Read the model definition and answer for the solid it produces. Units are mm, in the model's axes. Round coordinates to 2 decimals unless told otherwise and drop trailing zeros. Order: outer loops, then holes, each group sorted by start corner. A loop starts at its lowest first (then second) coordinate and runs counter-clockwise, first axis right, second up. Notation, with made-up numbers: (49, 68.5) - (103, 68.5) arc R18 cw to (103, 74.5) - close; hole circle Ø11 at (43, 33). An arc over 180 degrees is marked (long way). Answer as a JSON object with one key per item and string values. Group by question number.
Q1. A cutting plane is placed at A-A on y = -17. Determine the outline of the cut face in (x, z).
Q2. A cutting plane is placed at B-B on x = -18. Determine the outline of the cut face in (y, z) (3 decimals).
Q3. A cutting plane is placed at C-C on z = -24. Determine the outline of the cut face in (x, y) (3 decimals), and give its area (3 significant figures).
Q4. Given pin 1 Ø10.5 at (y, z) = (-7.5, 3) entering from +X; pin 2 Ø2.5 at (x, y) = (-34.5, -12) entering from -Z; pin 3 Ø2.5 at (x, y) = (-34, -14.5) entering from +Z, each flat-ended and moving along its own axis, determine where each tip first touches the part or whether it passes through.
Q5. Consider line 1 (Z direction, x = -45.5, y = -2.75); line 2 (Y direction, x = -12, z = 80) (3 decimals); line 3 (X direction, y = -7.5, z = 2). Determine where each line is inside the solid, lowest interval first.
```python
from build123d import *

# Parameters (mm, degrees)
F0_W        = 101.6
F0_H        = 279.4
F1_DEPTH    = 3.175
F2_W        = 3.175
F2_H        = 12.99972
F3_DEPTH    = 16.27124
F2_W_2      = 14.77137
F4_DEPTH    = 25.4
F5_T1_DEPTH = 12.99972
F7_D        = 6.10108


# Not quite as in the source:
# - a fillet or chamfer that OpenCascade refuses, or shapes differently, is made with other operations: its cross-section is extruded or revolved along the edge and cut away or added


with BuildPart() as f1:
    # F0 (on Front) → F1 (new body)
    with BuildSketch(Plane.XZ):
        Rectangle(F0_W, F0_H)
    extrude(amount=F1_DEPTH)

    # F2 (on face) → F3 (join)
    with BuildSketch(Plane.XZ.offset(3.175)):
        with Locations((34.44113, 0)):
            Rectangle(F2_W, F2_H)
        with Locations((-34.44113, 0)):
            Rectangle(F2_W, F2_H)
    extrude(amount=F3_DEPTH)

    # F2 (on face) → F4 (cut)
    with BuildSketch(Plane.XZ.offset(3.175)):
        with Locations((43.414315, 0)):
            Rectangle(F2_W_2, F2_H)
        with Locations((-43.414315, 0)):
            Rectangle(F2_W_2, F2_H)
    extrude(amount=-F4_DEPTH, mode=Mode.SUBTRACT)

    # F5: fillet of radius 5.08 on 2 edges, made by hand

    # F5_s2 → F5_t1 (cut)
    with BuildSketch(Plane.XY.offset(-6.49986)):
        with BuildLine():
            ThreePointArc((30.94863, 0), (34.5407324484, -1.4878975516), (36.02863, -5.08))
            Line((36.02863, -5.08), (36.02863, 0))
            Line((36.02863, 0), (30.94863, 0))
        make_face()
        with BuildLine():
            ThreePointArc((-30.94863, 0), (-34.5407324484, -1.4878975516), (-36.02863, -5.08))
            Line((-36.02863, -5.08), (-36.02863, 0))
            Line((-36.02863, 0), (-30.94863, 0))
        make_face()
    extrude(amount=F5_T1_DEPTH, mode=Mode.SUBTRACT)

    # F7 (through all)
    with Locations(Plane.YZ.offset(36.02863)):
        with Locations((-11.31062, 0)):
            Hole(F7_D / 2)


solid = f1.part
```
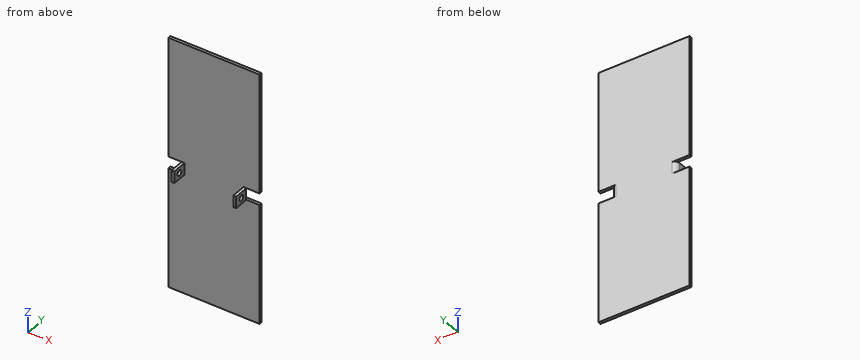
Result set:
{
 "1": {"outline": "(-36.03, -6.5) - (-32.85, -6.5) - (-32.85, 6.5) - (-36.03, 6.5) - close; (32.85, -6.5) - (36.03, -6.5) - (36.03, 6.5) - (32.85, 6.5) - close"},
 "2": {"outline": "(-3.175, -139.7) - (0, -139.7) - (0, 139.7) - (-3.175, 139.7) - close"},
 "3": {"outline": "(-50.8, -3.175) - (50.8, -3.175) - (50.8, 0) - (-50.8, 0) - close", "area": "323 mm²"},
 "4": {"pin 1": "stops at x = 36.03", "pin 2": "stops at z = -6.5", "pin 3": "stops at z = 6.5"},
 "5": {"line 1": "z = -139.7 to -6.5, 6.5 to 139.7", "line 2": "y = -3.175 to 0", "line 3": "x = -36.03 to -32.85, 32.85 to 36.03"}
}
